Check sheet for the drawn part. Datum: minimum x, y, z corner. Units: mm. Round coordinates to 2 decimals unless told otherwise and drop trailing zeros. Loops run counter-clockwise (first coordinate to the right, second up) from the corner with the lowest first, then second, coordinate; pieces in that order, holes last. Notation, with made-up numbers: (2.5, 38) - (42.5, 38) arc R13 ccw to (42.5, 42) - close; hole circle Ø10 at (27, -8.75). An arc over 180 degrees is marked (long way). Use CSV: the item, a comma, the result in double quotes.
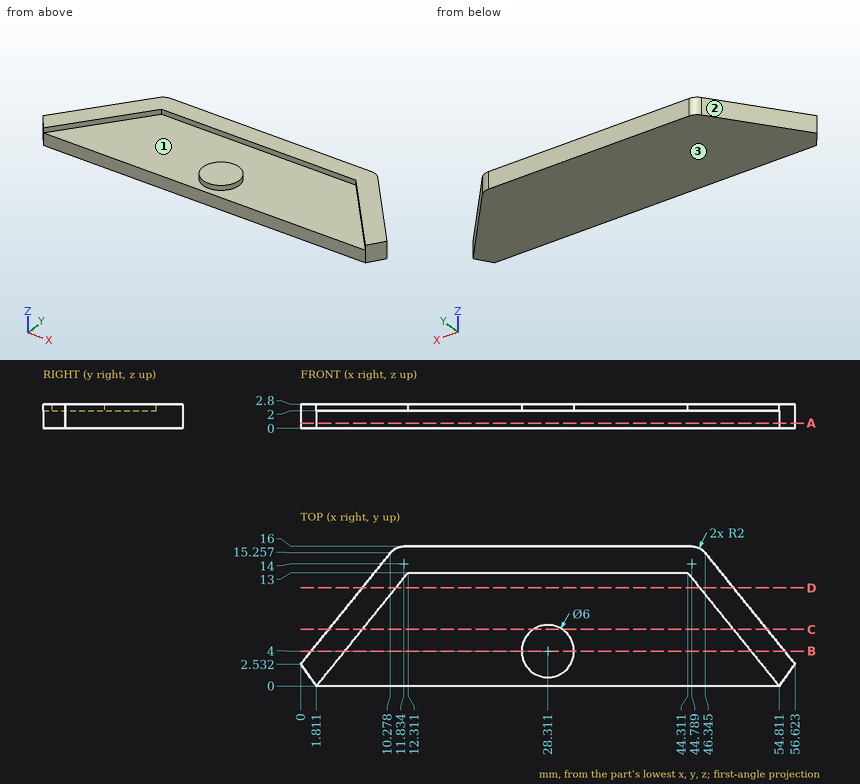
1) Cross-section at B-B, the plane y = 4. Record the cut outline in (x, z) (1 decimal).
Returned:
outline,"(1.2, 0) - (55.4, 0) - (55.4, 2.8) - (51.6, 2.8) - (51.6, 2) - (31.3, 2) - (31.3, 2.8) - (25.3, 2.8) - (25.3, 2) - (5, 2) - (5, 2.8) - (1.2, 2.8) - close"
2) Gauge pin test, flat ends, axial feed: pin 1 Ø8 at (x, y) = (20.5, 7) entering from +Z; pin 2 Ø0.9 at (x, z) = (26.5, 2.5) entering from -Y. Record the tip position at first contact, or that the pin passes through.
Returned:
pin 1,"stops at z = 2"
pin 2,"stops at y = 1.33"
3) Thickness scan on probe 1 along Z at (x, y) = (51, 4.5); probe 2 along Y at (x, z) = (42, 2.35); probe 3 along X at (y, z) = (6.75, 2.15) (1 decimal). Record the ranges inside material, lowest first. Write a range as [from, to].
Returned:
probe 1,"z = [0, 2]"
probe 2,"y = [13, 16]"
probe 3,"x = [3.4, 7.3], [27.1, 29.5], [49.4, 53.2]"
4) Cross-section at A-A, the plane z = 0.6. Record the cut outline in (x, y) (1 decimal).
Returned:
outline,"(0, 2.5) - (1.8, 0) - (54.8, 0) - (56.6, 2.5) - (46.3, 15.3) arc R2 ccw to (44.8, 16) - (11.8, 16) arc R2 ccw to (10.3, 15.3) - close"
5) Mould release check, pull along X, two halves, no side actions. Record for the marked faces 1, 2 and 3: +X half, -X half, draft (parallel to the pull), parting line (faces both ways), or undercut.
Returned:
face 1,"undercut"
face 2,"-X half"
face 3,"draft"
6) Cross-section at D-D, the plane y = 11.25. Record the cut outline in (x, z) (1 decimal).
Returned:
outline,"(7, 0) - (49.6, 0) - (49.6, 2.8) - (45.7, 2.8) - (45.7, 2) - (10.9, 2) - (10.9, 2.8) - (7, 2.8) - close"
7) Cross-section at C-C, the plane y = 6.5. Record the cut outline in (x, z) (1 decimal), then the cut area to 3 significant figures.
Returned:
outline,"(3.2, 0) - (53.4, 0) - (53.4, 2.8) - (49.6, 2.8) - (49.6, 2) - (30, 2) - (30, 2.8) - (26.7, 2.8) - (26.7, 2) - (7.1, 2) - (7.1, 2.8) - (3.2, 2.8) - close"
area,"109 mm²"
